Could you check a few things on this model? Use its own coordinates, in mm. Face numbers are marked on the shaded views. A direction names the side the tool comes from. Coordinates: 2 decimals unless noted, no trailing zeros. Order: outer loops, then holes, each group sorted by start corner. A loop starts at its lowest first (then second) coordinate and runs counter-clockwise, first axis right, second up. Notation, with made-up numbers: (82.5, 51.25) -> (92.5, 51.25) arc R28 ccw to (92.5, 75.25) -> close; hole circle Ø6 at (26.25, 75.25). An arc over 180 degrees is marked (long way). Use a Markdown table: item, result. Add a question column.
1) Which directions (+Z, -Z, +X, -X, +Y, -Y) give clear straight access to the entire face, cutting with the end or side of a thin tool? Please do the marked faces 1, 2 and 3.
2) If we section it at A-A (x = 42.5): Write out the boundary of the cut face in (y, z).
3) If I drill on L1, parallel to Y at x = 85.5, z = -11; L2, parallel to Y at x = 53, z = -101, over which ranges is the centre line in solid material (lowest first)? Write a range as [from, to].
4) If we section it at C-C (z = -72): Write out the boundary of the cut face in (x, y).
5) Will these pins go through, and if not, where does the flat tip stop? pin 1 Ø4 at (x, z) = (15, -4) entering from +Y; pin 2 Ø1.7 at (x, y) = (34.5, -12) entering from -Z; pin 3 Ø4.5 at (x, y) = (66, 62) entering from +Z.
6) If we section it at B-B (z = -101): Write out the boundary of the cut face in (x, y), plus the area to 3 significant figures.
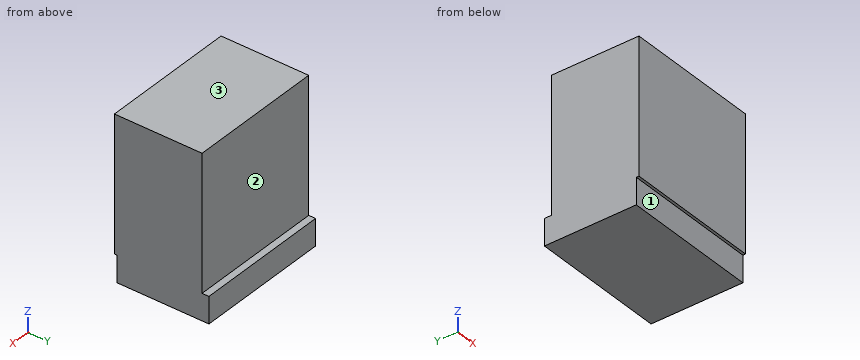
```python
from build123d import *

# Parameters (mm, degrees)
SCROD_AND_CARRIERS_AND_HV_DEPTH      = 57.8026
SCROD_AND_CARRIERS_AND_HV_DEPTH_BACK = 13
SKETCH1_W                            = 110
SKETCH1_H                            = 108.6724
SKETCH2_W                            = 110
SKETCH2_H                            = 74.2
PMT_ASSEMBLY_DEPTH                   = 21.4016


with BuildPart() as part:
    # Sketch1 → SCROD-and-carriers-and-HV (new, two sides: drawn at the far end of the back side and taken through both)
    with BuildSketch(Plane(origin=(0, 0, 0), x_dir=(1, 0, 0), z_dir=(0, 1, 0)).offset(-SCROD_AND_CARRIERS_AND_HV_DEPTH_BACK)):
        with Locations((55, 39.3362)):
            Rectangle(SKETCH1_W, SKETCH1_H)
    extrude(amount=SCROD_AND_CARRIERS_AND_HV_DEPTH + SCROD_AND_CARRIERS_AND_HV_DEPTH_BACK)

    # Sketch2 → pmt-assembly (add)
    with BuildSketch(Plane(origin=(0, 0, -93.6724), x_dir=(-1, 0, 0), z_dir=(0, 0, -1))):
        with Locations((-55, 26.2526)):
            Rectangle(SKETCH2_W, SKETCH2_H)
    extrude(amount=PMT_ASSEMBLY_DEPTH)


solid = part.part
```
Answer sheet:
| question | item | result |
|---|---|---|
| 1 | face 1 | -Z, +X, -X, -Y |
| 1 | face 2 | +Z, +X, -X, +Y |
| 1 | face 3 | +Z, +X, -X, +Y, -Y |
| 2 | outline | (-13, -93.67) -> (-10.85, -93.67) -> (-10.85, -115.07) -> (63.35, -115.07) -> (63.35, -93.67) -> (57.8, -93.67) -> (57.8, 15) -> (-13, 15) -> close |
| 3 | L1 | [-13, 57.8] |
| 3 | L2 | [-10.85, 63.35] |
| 4 | outline | (0, -13) -> (110, -13) -> (110, 57.8) -> (0, 57.8) -> close |
| 5 | pin 1 | y = 57.8 |
| 5 | pin 2 | z = -93.67 |
| 5 | pin 3 | z = -93.67 |
| 6 | outline | (0, -10.85) -> (110, -10.85) -> (110, 63.35) -> (0, 63.35) -> close |
| 6 | area | 8,160 mm2 |
